Check sheet for the modelled part. Datum: model origin and axes. Units: mm. A direction names the side the tool comes from. Round coordinates to 2 decimals unless told otherwise and drop trailing zeros. Loops run counter-clockwise (first coordinate to the right, second up) from the corner with the lowest first, then second, coordinate; pieces in that order, holes last. Notation, with made-up numbers: (48.25, 21.5) - (69.25, 21.5) arc R18 cw to (69.25, 34.5) - close; hole circle Ø11 at (54.25, -37.5). An arc over 180 degrees is marked (long way). Answer in a Markdown table with one row per item. Add a question column.
(1) Access from +Z, -Z, +X, -X, +Y, -Y to the whole of each face (thin tool, end or side, straight path). Record for faces 1 (the flat face through (3, 17, 0)), 2 (the flat face through (0, 12.4, -1.9)), 3 (the flat face through (1.73, 9, -3)), 4 (the flat face through (11, 1.73, 3)).
(2) Mould release check, pull along X, two halves, no side actions. Record for faces 5 (the cylindrical face through (2.43, 19.4, 0.13)), 6 (the flat face through (12.1, 0, 2.1)), 7 (the cylindrical face through (7.43, 0.85, 1.06)): +X half, -X half, draft (parallel to the pull), parting line (faces both ways), or undercut.
(3) Cross-section at D-D on y = 14.25. Enter the section's corners in (x, z).
(4) Cross-section at A-A on y = 10. Enter the section's corners in (x, z), then the cut area to 3 significant figures.
(5) Cross-section at B-B on z = 0. Enter the section's corners in (x, y).
(6) Gauge pin test, flat ends, axial feed: pin 1 (2 mm diameter, centred on x = 4.5, y = 13.5, fed in from -Z); pin 2 (9 mm diameter, centred on x = 10, z = 0, fed in from +Y); pin 3 (6.5 mm diameter, centred on x = 12.5, z = 3, fed in from +Y); pin 4 (6.5 mm diameter, centred on y = 10.5, z = -2.5, fed in from +X). Record the tip position at first contact, or that the pin passes through.
(7) Thickness scan on line 1 along Z through (x, y) = (2.4, 10); line 2 along X through (y, z) = (1, 0); line 3 along Z through (x, y) = (10, 0.55). Record the ranges inside material, lowest first.
from build123d import *

# Parameters (mm, degrees)
BOSS_EXTRUDE1_DEPTH     = 9
SKETCH2_R               = 2.78
CUT_EXTRUDE1_DEPTH      = 21
SKETCH3_R               = 2.78
CUT_EXTRUDE2_DEPTH      = 21
SKETCH6_R               = 6.35
CUT_EXTRUDE3_DEPTH      = 18
CUT_EXTRUDE3_DEPTH_BACK = 1.27
SKETCH7_R               = 6.35
CUT_EXTRUDE4_DEPTH      = 18
CUT_EXTRUDE4_DEPTH_BACK = 1.27


with BuildPart() as part:
    # Sketch1 → Boss-Extrude1 (new body, symmetric)
    with BuildSketch(Plane.XY):
        with BuildLine():
            Line((0, 0), (20, 0))
            Line((20, 0), (20, 1))
            ThreePointArc((20, 1), (19.414213562, 2.414213562), (18, 3))
            Line((18, 3), (5, 3))
            ThreePointArc((5, 3), (3.585786438, 3.585786438), (3, 5))
            Line((3, 5), (3, 18))
            ThreePointArc((3, 18), (2.414213562, 19.414213562), (1, 20))
            Line((1, 20), (0, 20))
            Line((0, 20), (0, 0))
        make_face()
    extrude(amount=BOSS_EXTRUDE1_DEPTH, both=True)

    # Sketch2 → Cut-Extrude1 (cut, through all)
    with BuildSketch(Plane(origin=(0, 0, 0), x_dir=(-1, 0, 0), z_dir=(0, -1, 0))):
        with Locations((-10, 0)):
            Circle(SKETCH2_R)
    extrude(amount=-CUT_EXTRUDE1_DEPTH, mode=Mode.SUBTRACT)

    # Sketch3 → Cut-Extrude2 (cut, through all)
    with BuildSketch(Plane.ZY):
        with Locations((0, 10)):
            Circle(SKETCH3_R)
    extrude(amount=-CUT_EXTRUDE2_DEPTH, mode=Mode.SUBTRACT)

    # Sketch6 → Cut-Extrude3 (cut, two sides)
    with BuildSketch(Plane(origin=(3, 0, 0), x_dir=(0, 0, -1), z_dir=(1, 0, 0))) as cut_extrude3_sk:
        with Locations((0, 10)):
            Circle(SKETCH6_R)
    extrude(amount=CUT_EXTRUDE3_DEPTH, mode=Mode.SUBTRACT)
    extrude(cut_extrude3_sk.sketch, amount=-CUT_EXTRUDE3_DEPTH_BACK, mode=Mode.SUBTRACT)

    # Sketch7 → Cut-Extrude4 (cut, two sides)
    with BuildSketch(Plane(origin=(0, 3, 0), x_dir=(1, 0, 0), z_dir=(0, 1, 0))) as cut_extrude4_sk:
        with Locations((10, 0)):
            Circle(SKETCH7_R)
    extrude(amount=CUT_EXTRUDE4_DEPTH, mode=Mode.SUBTRACT)
    extrude(cut_extrude4_sk.sketch, amount=-CUT_EXTRUDE4_DEPTH_BACK, mode=Mode.SUBTRACT)


solid = part.part
Answers:
| question | item | result |
|---|---|---|
| 1 | face 1 | +Z, -Z, +X, +Y |
| 1 | face 2 | +Z, -Z, -X, +Y, -Y |
| 1 | face 3 | +X |
| 1 | face 4 | +Y |
| 2 | face 5 | +X half |
| 2 | face 6 | draft |
| 2 | face 7 | undercut |
| 3 | outline | (0, -9) - (3, -9) - (3, -4.72) - (1.73, -4.72) - (1.73, 4.72) - (3, 4.72) - (3, 9) - (0, 9) - close |
| 4 | outline | (0, -9) - (3, -9) - (3, -6.35) - (1.73, -6.35) - (1.73, -2.78) - (0, -2.78) - close; (0, 2.78) - (1.73, 2.78) - (1.73, 6.35) - (3, 6.35) - (3, 9) - (0, 9) - close |
| 4 | area | 28.3 mm^2 |
| 5 | outline | (0, 0) - (7.22, 0) - (7.22, 1.73) - (3.65, 1.73) - (3.65, 3.52) arc R2 cw to (3.52, 3.65) - (1.73, 3.65) - (1.73, 7.22) - (0, 7.22) - close; (0, 12.78) - (1.73, 12.78) - (1.73, 16.35) - (3, 16.35) - (3, 18) arc R2 ccw to (1, 20) - (0, 20) - close; (12.78, 0) - (20, 0) - (20, 1) arc R2 ccw to (18, 3) - (16.35, 3) - (16.35, 1.73) - (12.78, 1.73) - close |
| 6 | pin 1 | passes through |
| 6 | pin 2 | stops at y = 1.73 |
| 6 | pin 3 | stops at y = 3 |
| 6 | pin 4 | stops at x = 1.73 |
| 7 | line 1 | z = -9 to -6.35, 6.35 to 9 |
| 7 | line 2 | x = 0 to 7.22, 12.78 to 20 |
| 7 | line 3 | z = -9 to -2.78, 2.78 to 9 |
